Design review of the part built by this model. Coordinates are the model's own, in mm. Face numbers are marked on the shaded views. A direction names the side the tool comes from. Round coordinates to 2 decimals unless told otherwise and drop trailing zeros. Loops run counter-clockwise (first coordinate to the right, second up) from the corner with the lowest first, then second, coordinate; pieces in that order, holes last. Notation, with made-up numbers: M -22,48.5 L 17,48.5 A10 cw 17,57.5 Z; hole C 75.5,-17 d1. An arc over 180 degrees is marked long. Use a Markdown table: item, result.
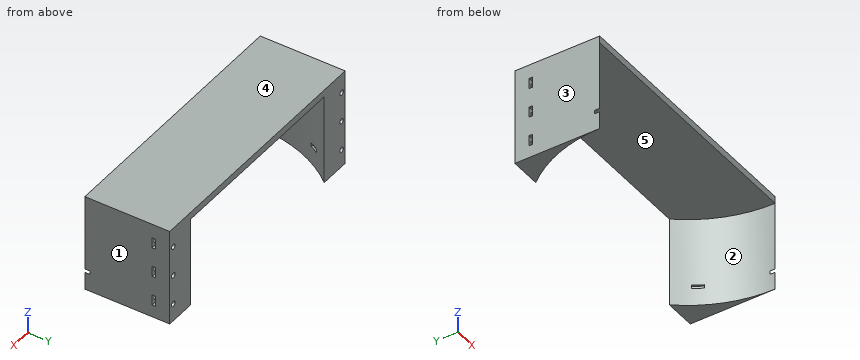
from build123d import *

# Parameters (mm, degrees)
BOX700_W               = 6
BOX700_H               = 8
BOX700_DEPTH           = 2
BOX700_PLACEMENT_ANGLE = 30
BOX701_W               = 6
BOX701_H               = 8
BOX701_DEPTH           = 2
BOX701_PLACEMENT_ANGLE = 60
BOX702_W               = 6
BOX702_H               = 8
BOX702_DEPTH           = 2
BOX703_W               = 6
BOX703_H               = 8
BOX703_DEPTH           = 2
BOX703_PLACEMENT_ANGLE = 120
BOX704_W               = 6
BOX704_H               = 8
BOX704_DEPTH           = 2
BOX704_PLACEMENT_ANGLE = 150
BOX705_W               = 6
BOX705_H               = 8
BOX705_DEPTH           = 2
BOX706_W               = 6
BOX706_H               = 8
BOX706_DEPTH           = 2
BOX706_PLACEMENT_ANGLE = 210
BOX707_W               = 6
BOX707_H               = 8
BOX707_DEPTH           = 2
BOX707_PLACEMENT_ANGLE = 240
BOX708_W               = 6
BOX708_H               = 8
BOX708_DEPTH           = 2
BOX709_W               = 6
BOX709_H               = 8
BOX709_DEPTH           = 2
BOX709_PLACEMENT_ANGLE = 60
BOX710_W               = 6
BOX710_H               = 8
BOX710_DEPTH           = 2
BOX710_PLACEMENT_ANGLE = 30
BOX699_W               = 6
BOX699_H               = 8
BOX699_DEPTH           = 2
BOX513_W               = 8
BOX513_H               = 2
BOX513_DEPTH           = 6
BOX514_W               = 8
BOX514_H               = 2
BOX514_DEPTH           = 6
BOX515_W               = 8
BOX515_H               = 2
BOX515_DEPTH           = 6
BOX516_W               = 8
BOX516_H               = 2
BOX516_DEPTH           = 6
BOX517_W               = 8
BOX517_H               = 2
BOX517_DEPTH           = 6
BOX512_W               = 8
BOX512_H               = 2
BOX512_DEPTH           = 6
CYLINDER1754_R         = 1.5
CYLINDER1754_DEPTH     = 50
CYLINDER1755_R         = 1.5
CYLINDER1755_DEPTH     = 50
CYLINDER1756_R         = 1.5
CYLINDER1756_DEPTH     = 50
CYLINDER1757_R         = 1.5
CYLINDER1757_DEPTH     = 50
CYLINDER1758_R         = 1.5
CYLINDER1758_DEPTH     = 50
CYLINDER1753_R         = 1.5
CYLINDER1753_DEPTH     = 50
BOX484_W               = 148
BOX484_H               = 26
BOX484_DEPTH           = 55
CYLINDER972_R          = 74
CYLINDER972_DEPTH      = 51
BOX482_W               = 148
BOX482_H               = 74
BOX482_DEPTH           = 55


with BuildPart() as krychle700:
    # Box700 → Box700 (new body)
    with BuildSketch(Plane.XY):
        with Locations((3, 4)):
            Rectangle(BOX700_W, BOX700_H)
    extrude(amount=BOX700_DEPTH)


with BuildPart() as krychle700_1:
    # Box700 placement: moved
    add(krychle700.part.moved(Location((34.901924, -66.451905, 39))).rotate(Axis((34.901924, -66.451905, 39), (0, 0, 1)), BOX700_PLACEMENT_ANGLE))


with BuildPart() as krychle701:
    # Box701 → Box701 (new body)
    with BuildSketch(Plane.XY):
        with Locations((3, 4)):
            Rectangle(BOX701_W, BOX701_H)
    extrude(amount=BOX701_DEPTH)


with BuildPart() as krychle701_1:
    # Box701 placement: moved
    add(krychle701.part.moved(Location((63.451905, -40.098076, 39))).rotate(Axis((63.451905, -40.098076, 39), (0, 0, 1)), BOX701_PLACEMENT_ANGLE))


with BuildPart() as krychle702:
    # Box702 → Box702 (new body)
    with BuildSketch(Plane(origin=(75, -3, 39), x_dir=(0, 1, 0), z_dir=(0, 0, 1))):
        with Locations((3, 4)):
            Rectangle(BOX702_W, BOX702_H)
    extrude(amount=BOX702_DEPTH)


with BuildPart() as krychle703:
    # Box703 → Box703 (new body)
    with BuildSketch(Plane.XY):
        with Locations((3, 4)):
            Rectangle(BOX703_W, BOX703_H)
    extrude(amount=BOX703_DEPTH)


with BuildPart() as krychle703_1:
    # Box703 placement: moved
    add(krychle703.part.moved(Location((66.451905, 34.901924, 39))).rotate(Axis((66.451905, 34.901924, 39), (0, 0, 1)), BOX703_PLACEMENT_ANGLE))


with BuildPart() as krychle704:
    # Box704 → Box704 (new body)
    with BuildSketch(Plane.XY):
        with Locations((3, 4)):
            Rectangle(BOX704_W, BOX704_H)
    extrude(amount=BOX704_DEPTH)


with BuildPart() as krychle704_1:
    # Box704 placement: moved
    add(krychle704.part.moved(Location((40.098076, 63.451905, 39))).rotate(Axis((40.098076, 63.451905, 39), (0, 0, 1)), BOX704_PLACEMENT_ANGLE))


with BuildPart() as krychle705:
    # Box705 → Box705 (new body)
    with BuildSketch(Plane(origin=(3, 75, 39), x_dir=(-1, 0, 0), z_dir=(0, 0, 1))):
        with Locations((3, 4)):
            Rectangle(BOX705_W, BOX705_H)
    extrude(amount=BOX705_DEPTH)


with BuildPart() as krychle706:
    # Box706 → Box706 (new body)
    with BuildSketch(Plane.XY):
        with Locations((3, 4)):
            Rectangle(BOX706_W, BOX706_H)
    extrude(amount=BOX706_DEPTH)


with BuildPart() as krychle706_1:
    # Box706 placement: moved
    add(krychle706.part.moved(Location((-34.901924, 66.451905, 39))).rotate(Axis((-34.901924, 66.451905, 39), (0, 0, 1)), BOX706_PLACEMENT_ANGLE))


with BuildPart() as krychle707:
    # Box707 → Box707 (new body)
    with BuildSketch(Plane.XY):
        with Locations((3, 4)):
            Rectangle(BOX707_W, BOX707_H)
    extrude(amount=BOX707_DEPTH)


with BuildPart() as krychle707_1:
    # Box707 placement: moved
    add(krychle707.part.moved(Location((-63.451905, 40.098076, 39))).rotate(Axis((-63.451905, 40.098076, 39), (0, 0, 1)), BOX707_PLACEMENT_ANGLE))


with BuildPart() as krychle708:
    # Box708 → Box708 (new body)
    with BuildSketch(Plane(origin=(-75, 3, 39), x_dir=(0, -1, 0), z_dir=(0, 0, 1))):
        with Locations((3, 4)):
            Rectangle(BOX708_W, BOX708_H)
    extrude(amount=BOX708_DEPTH)


with BuildPart() as krychle709:
    # Box709 → Box709 (new body)
    with BuildSketch(Plane.XY):
        with Locations((3, 4)):
            Rectangle(BOX709_W, BOX709_H)
    extrude(amount=BOX709_DEPTH)


with BuildPart() as krychle709_1:
    # Box709 placement: moved
    add(krychle709.part.moved(Location((-66.451905, -34.901924, 39))).rotate(Axis((-66.451905, -34.901924, 39), (0, 0, -1)), BOX709_PLACEMENT_ANGLE))


with BuildPart() as krychle710:
    # Box710 → Box710 (new body)
    with BuildSketch(Plane.XY):
        with Locations((3, 4)):
            Rectangle(BOX710_W, BOX710_H)
    extrude(amount=BOX710_DEPTH)


with BuildPart() as krychle710_1:
    # Box710 placement: moved
    add(krychle710.part.moved(Location((-40.098076, -63.451905, 39))).rotate(Axis((-40.098076, -63.451905, 39), (0, 0, -1)), BOX710_PLACEMENT_ANGLE))


with BuildPart() as compound888:
    # Box699 → Box699 (new body)
    with BuildSketch(Plane(origin=(-3, -75, 39), x_dir=(1, 0, 0), z_dir=(0, 0, 1))):
        with Locations((3, 4)):
            Rectangle(BOX699_W, BOX699_H)
    extrude(amount=BOX699_DEPTH)

    # Compound888: union Krychle700, Krychle701, Krychle702, Krychle703, Krychle704, Krychle705, Krychle706, Krychle707, Krychle708, Krychle709, Krychle710
    add(krychle700_1.part)
    add(krychle701_1.part)
    add(krychle702.part)
    add(krychle703_1.part)
    add(krychle704_1.part)
    add(krychle705.part)
    add(krychle706_1.part)
    add(krychle707_1.part)
    add(krychle708.part)
    add(krychle709_1.part)
    add(krychle710_1.part)


with BuildPart() as krychle513:
    # Box513 → Box513 (new body)
    with BuildSketch(Plane(origin=(67, 38, 36), x_dir=(1, 0, 0), z_dir=(0, 0, 1))):
        with Locations((4, 1)):
            Rectangle(BOX513_W, BOX513_H)
    extrude(amount=BOX513_DEPTH)


with BuildPart() as krychle514:
    # Box514 → Box514 (new body)
    with BuildSketch(Plane(origin=(67, 38, 70), x_dir=(1, 0, 0), z_dir=(0, 0, 1))):
        with Locations((4, 1)):
            Rectangle(BOX514_W, BOX514_H)
    extrude(amount=BOX514_DEPTH)


with BuildPart() as krychle515:
    # Box515 → Box515 (new body)
    with BuildSketch(Plane(origin=(-75, 38, 70), x_dir=(1, 0, 0), z_dir=(0, 0, 1))):
        with Locations((4, 1)):
            Rectangle(BOX515_W, BOX515_H)
    extrude(amount=BOX515_DEPTH)


with BuildPart() as krychle516:
    # Box516 → Box516 (new body)
    with BuildSketch(Plane(origin=(-75, 38, 53), x_dir=(1, 0, 0), z_dir=(0, 0, 1))):
        with Locations((4, 1)):
            Rectangle(BOX516_W, BOX516_H)
    extrude(amount=BOX516_DEPTH)


with BuildPart() as krychle517:
    # Box517 → Box517 (new body)
    with BuildSketch(Plane(origin=(67, 38, 53), x_dir=(1, 0, 0), z_dir=(0, 0, 1))):
        with Locations((4, 1)):
            Rectangle(BOX517_W, BOX517_H)
    extrude(amount=BOX517_DEPTH)


with BuildPart() as compound530:
    # Box512 → Box512 (new body)
    with BuildSketch(Plane(origin=(-75, 38, 36), x_dir=(1, 0, 0), z_dir=(0, 0, 1))):
        with Locations((4, 1)):
            Rectangle(BOX512_W, BOX512_H)
    extrude(amount=BOX512_DEPTH)

    # Compound530: union Krychle513, Krychle514, Krychle515, Krychle516, Krychle517
    add(krychle513.part)
    add(krychle514.part)
    add(krychle515.part)
    add(krychle516.part)
    add(krychle517.part)


with BuildPart() as obj1:
    # Cylinder1754 → Cylinder1754 (new body)
    with BuildSketch(Plane(origin=(71, 80, 39), x_dir=(1, 0, 0), z_dir=(0, -1, 0))):
        Circle(CYLINDER1754_R)
    extrude(amount=CYLINDER1754_DEPTH)


with BuildPart() as obj2:
    # Cylinder1755 → Cylinder1755 (new body)
    with BuildSketch(Plane(origin=(-71, 80, 39), x_dir=(1, 0, 0), z_dir=(0, -1, 0))):
        Circle(CYLINDER1755_R)
    extrude(amount=CYLINDER1755_DEPTH)


with BuildPart() as obj3:
    # Cylinder1756 → Cylinder1756 (new body)
    with BuildSketch(Plane(origin=(71, 80, 73), x_dir=(1, 0, 0), z_dir=(0, -1, 0))):
        Circle(CYLINDER1756_R)
    extrude(amount=CYLINDER1756_DEPTH)


with BuildPart() as obj4:
    # Cylinder1757 → Cylinder1757 (new body)
    with BuildSketch(Plane(origin=(-71, 80, 56), x_dir=(1, 0, 0), z_dir=(0, -1, 0))):
        Circle(CYLINDER1757_R)
    extrude(amount=CYLINDER1757_DEPTH)


with BuildPart() as obj5:
    # Cylinder1758 → Cylinder1758 (new body)
    with BuildSketch(Plane(origin=(71, 80, 56), x_dir=(1, 0, 0), z_dir=(0, -1, 0))):
        Circle(CYLINDER1758_R)
    extrude(amount=CYLINDER1758_DEPTH)


with BuildPart() as compound887:
    # Cylinder1753 → Cylinder1753 (new body)
    with BuildSketch(Plane(origin=(-71, 80, 73), x_dir=(1, 0, 0), z_dir=(0, -1, 0))):
        Circle(CYLINDER1753_R)
    extrude(amount=CYLINDER1753_DEPTH)

    # Compound887: union obj1, obj2, obj3, obj4, obj5
    add(obj1.part)
    add(obj2.part)
    add(obj3.part)
    add(obj4.part)
    add(obj5.part)


with BuildPart() as krychle484:
    # Box484 → Box484 (new body)
    with BuildSketch(Plane(origin=(-74, 48, 29), x_dir=(1, 0, 0), z_dir=(0, 0, 1))):
        with Locations((74, 13)):
            Rectangle(BOX484_W, BOX484_H)
    extrude(amount=BOX484_DEPTH)


with BuildPart() as obj6:
    # Cylinder972 → Cylinder972 (new body)
    with BuildSketch(Plane.XY.offset(29)):
        Circle(CYLINDER972_R)
    extrude(amount=CYLINDER972_DEPTH)


with BuildPart() as cut520:
    # Box482 → Box482 (new body)
    with BuildSketch(Plane(origin=(-74, 0, 29), x_dir=(1, 0, 0), z_dir=(0, 0, 1))):
        with Locations((74, 37)):
            Rectangle(BOX482_W, BOX482_H)
    extrude(amount=BOX482_DEPTH)

    # Cut451: cut obj6
    add(obj6.part, mode=Mode.SUBTRACT)

    # Cut452: cut Krychle484
    add(krychle484.part, mode=Mode.SUBTRACT)

    # Cut518: cut Compound887
    add(compound887.part, mode=Mode.SUBTRACT)

    # Cut519: cut Compound530
    add(compound530.part, mode=Mode.SUBTRACT)

    # Cut520: cut Compound888
    add(compound888.part, mode=Mode.SUBTRACT)


solid = cut520.part
1. Take a section at C-C on y = 20. Give the boundary of the cut face in (x, z).
Check values:
| item | result |
|---|---|
| outline | M -74,29 L -71.25,29 L -71.25,80 L 71.25,80 L 71.25,29 L 74,29 L 74,84 L -74,84 Z |
2. Take a section at B-B on z = 64.5. Give the boundary of the cut face in (x, y), and give its area (3 significant figures).
Check values:
| item | result |
|---|---|
| outline | M -74,0 A74 cw -56.32,48 L -74,48 Z; M 56.32,48 A74 cw 74,0 L 74,48 Z |
| area | 536 mm² |
3. Wall thickness on line 1 along Z through (x, y) = (-71, 43); line 2 along X through (y, z) = (35, 56); line 3 along X through (y, z) = (33, 56): over which ranges is each line inside the solid? List them lowest first. Write a range as from..to.
Check values:
| item | result |
|---|---|
| line 1 | z = 29..37.5, 40.5..54.5, 57.5..71.5, 74.5..84 |
| line 2 | x = -74..-72.5, -69.5..-65.2, 65.2..69.5, 72.5..74 |
| line 3 | x = -74..-72.5, -69.5..-66.23, 66.23..69.5, 72.5..74 |
4. Machinability: for the marked faces 4 and 5, which of the approach directions +Z, -Z, +X, -X, +Y, -Y give a long, thin tool a straight path to every point of the face, cutting with its end or side? Answer none if there is none.
Check values:
| item | result |
|---|---|
| face 4 | +Z, +X, -X, +Y, -Y |
| face 5 | -Z, -Y |
5. Insertion check: pin 1 (24 mm diameter, centred on x = 32, y = 31.5, fed in from -Z); pin 2 (2.5 mm diameter, centred on x = -71, z = 39, fed in from +Y); pin 3 (0.6 mm diameter, centred on y = 39.5, z = 55.5, fed in from +X). Each pin has a flat end and moves straight along its axis. Give the tip position at first contact, or say it passes through.
Check values:
| item | result |
|---|---|
| pin 1 | stops at z = 80 |
| pin 2 | stops at y = 30 |
| pin 3 | stops at x = 67 |
6. Take a section at A-A on z = 56. Count the separate pieces of the cut face and the enclosed holes in it, and give its area (3 significant figures).
Check values:
| item | result |
|---|---|
| separate pieces | 4 |
| enclosed holes | 0 |
| area | 412 mm² |
7. The part is to be moulded in two halves that separate along X. For the marked faces 1, 2 and 3, say which applies: pulls with the +X half, pulls with the -X half, needs draft (parallel to the pull), parting line crosses it, or undercut.
Check values:
| item | result |
|---|---|
| face 1 | pulls with the +X half |
| face 2 | undercut |
| face 3 | pulls with the -X half |
8. Take a section at D-D on x = 21.5. Give the boundary of the cut face in (y, z), and give its area (3 significant figures).
Check values:
| item | result |
|---|---|
| outline | M 0,80 L 48,80 L 48,84 L 0,84 Z |
| area | 192 mm² |
